Here's how the part is built. I have some questions about the finished solid (model axes, mm). A direction names the side the tool comes from. Round coordinates to 2 decimals unless told otherwise and drop trailing zeros. Order: outer loops, then holes, each group sorted by start corner. A loop starts at its lowest first (then second) coordinate and runs counter-clockwise, first axis right, second up. Notation, with made-up numbers: M 68,86 L 93,86 A16 cw 93,104 Z; hole C 25,-24 d6. An arc over 180 degrees is marked long. Write item = value, one per line. Start each with the question number.
Item 1: For faces 5 (the face through (0.067, 5.525, 3.131)), 6 (the face through (-4.762, -8, 1)), which set-ups out of +Z, -Z, +X, -X, +Y, -Y let a thin tool reach every point of the face, with its end or its side?
Item 2: I'm going to push flat-ended pins straight in: P1, Ø1.5, axis at x = -0.5, y = -21, coming from the -Z side; P2, Ø3, axis at x = 3, y = 10, coming from the +Z side; P3, Ø2, axis at x = 4, z = -8.5, coming from the -Y side. Where does each tip first touch, or does it pass through?
Item 3: I want a section at D-D, the plane z = 8. List the corners of the cut face in (x, y) for me.
Item 4: Please list where these lines run through material, in increasing order: L1, parallel to Z at x = -2.5, y = 7; L2, parallel to Z at x = 2, y = 32; L3, parallel to Z at x = 3.25, y = 30.5.
Item 5: We'd pull the mould along Y, two halves only. Please class faces 1 (the face through (0.067, -5.474, 3.219)), 2 (the face through (4.762, -8, 1)), 3 (the face through (0, 0, -6.35)), 4 (the face through (0.067, 10.967, -34.826)): pulls with the +Y half, pulls with the -Y half, needs draft (parallel to the pull), parting line crosses it, or undercut.
Item 6: I want a section at A-A, the plane y = 0. List the corners of the cut face in (x, z) for me, plus the area to 3 significant figures.
Item 7: I want a section at C-C, the plane y = 32. List the corners of the cut face in (x, z) for me.
```python
from build123d import *

# Parameters (mm, degrees)
SKETCH2_R           = 36.5125
BOSS_EXTRUDE1_DEPTH = 4.7625


with BuildPart() as part:
    # Sketch2 → Boss-Extrude1 (new body, symmetric)
    with BuildSketch(Plane(origin=(0, 0, 0), x_dir=(0, 0, -1), z_dir=(1, 0, 0))):
        Circle(SKETCH2_R)
        Polygon((0, 7.332348419), (-6.35, 3.666174209), (-6.35, -3.666174209), (0, -7.332348419), (6.35, -3.666174209), (6.35, 3.666174209), align=None, mode=Mode.SUBTRACT)
    extrude(amount=BOSS_EXTRUDE1_DEPTH, both=True)


solid = part.part
```
Filled in:
q1.face_5 = +X, -X
q1.face_6 = +Z, -Z, -X, +Y, -Y
q2.P1 = -30.38
q2.P2 = 35.51
q2.P3 = -35.73
q3.outline = M -4.76,-35.63 L 4.76,-35.63 L 4.76,35.63 L -4.76,35.63 Z
q4.L1 = -35.84 to -0.58, 0.58 to 35.84
q4.L2 = -17.58 to 17.58
q4.L3 = -20.07 to 20.07
q5.face_1 = undercut
q5.face_2 = needs draft
q5.face_3 = undercut
q5.face_4 = parting line crosses it
q6.outline = M -4.76,-36.51 L 4.76,-36.51 L 4.76,-6.35 L -4.76,-6.35 Z; M -4.76,6.35 L 4.76,6.35 L 4.76,36.51 L -4.76,36.51 Z
q6.area = 575 mm^2
q7.outline = M -4.76,-17.58 L 4.76,-17.58 L 4.76,17.58 L -4.76,17.58 Z
